Here's how the part is built. I have some questions about the finished solid (model axes, mm). A direction names the side the tool comes from. Give positions to 0.01 mm unless a question says otherwise; leave off trailing zeros. Loops run counter-clockwise (first coordinate to the right, second up) from the corner with the lowest first, then second, coordinate; pieces in that order, holes last. Notation, with made-up numbers: (4, -35.75) -> (47, -35.75) arc R13 ccw to (47, -23.75) -> close; hole circle Ø4 at (7, 39.25). An arc over 180 degrees is marked (long way). Answer in a Markdown table with one row per item. Add a question column.
Item 1: If we section it at C-C (x = 69.5): Write out the boundary of the cut face in (y, z), then the cut area to 3 significant figures.
Item 2: For P1, Ø2, axis at x = 22, z = 36, coming from the +Y side; P2, Ø19, axis at x = 15.5, y = -41.5, coming from the +Z side (3 decimals); P3, Ø20.5, axis at y = 11, z = 26.5, coming from the -X side (3 decimals), each with a flat end and sliding along its axis, tell me the tip position at first contact or that it passes through.
Item 3: If we section it at B-B (y = -44): Write out the boundary of the cut face in (x, z) (3 decimals), then the cut area to 3 significant figures.
Item 4: If we section it at A-A (z = 1): Write out the boundary of the cut face in (x, y) (3 decimals), then the cut area to 3 significant figures.
Item 5: Which directions (+Z, -Z, +X, -X, +Y, -Y) give clear straight access to the entire face, cutting with the end or side of a thin tool? Please do faces 1 (the face through (-1, -1, -9.525)), 2 (the face through (63, 0, 44.542)), 3 (the face through (26.035, 13, 27)), 4 (the face through (48, 25.4, 46)), 5 (the face through (21, -25.4, 35)).
Item 6: If I drill on line 1 (Z direction, x = 65.5, y = -13); line 2 (Y direction, x = 63.5, z = 45.5); line 3 (Y direction, x = 16, z = 33), over which ranges is the centre line in solid material (lowest first)?
```python
from build123d import *

# Parameters (mm, degrees)
F1_DEPTH = 63.5
F0_W     = 25.4
F0_H     = 15.24
F2_DEPTH = 25.4
F3_DEPTH = 25.4
F4_R     = 6.35


with BuildPart() as f1:
    # F0 (on Front) → F1 (new body, symmetric)
    with BuildSketch(Plane.XZ):
        Polygon((41.275, -9.525), (41.275, 9.525), (26.035, 9.525), (-41.275, 9.525), (-41.275, -9.525), align=None)
    extrude(amount=F1_DEPTH, both=True)

    # F0 (on Front) → F2 (join, symmetric)
    with BuildSketch(Plane.XZ):
        with BuildLine():
            Line((26.035, 9.525), (41.275, 9.525))
            Line((41.275, 9.525), (41.275, 43.0532871165))
            ThreePointArc((41.275, 43.0532871165), (41.710954306, 44.1057739147), (42.7634411042, 44.5417282207))
            Line((42.7634411042, 44.5417282207), (58.6539360017, 44.5417282207))
            Line((58.6539360017, 44.5417282207), (58.6539360017, 59.7817282207))
            Line((58.6539360017, 59.7817282207), (42.7634411042, 59.7817282207))
            add(Edge.make_bspline(
                [(42.7634411042, 59.7817282207), (40.0314907438, 59.0712143993), (37.3116085618, 58.3664493175), (34.6130178648, 57.6618922106)],
                knots=[0, 0, 0, 0, 6.2650251323, 6.2650251323, 6.2650251323, 6.2650251323], degree=3))
            ThreePointArc((34.6130178648, 57.6618922106), (28.3380361374, 51.5237318109), (26.035, 43.0532871165))
            Line((26.035, 43.0532871165), (26.035, 9.525))
        make_face()
        with Locations((71.3539360017, 52.1617282207)):
            Rectangle(F0_W, F0_H)
    extrude(amount=F2_DEPTH, both=True)

    # F0 (on Front) → F3 (join)
    with BuildSketch(Plane.XZ):
        with BuildLine():
            Line((-41.275, 9.525), (26.035, 9.525))
            Line((26.035, 9.525), (26.035, 43.0532871165))
            ThreePointArc((26.035, 43.0532871165), (28.3380361374, 51.5237318109), (34.6130178648, 57.6618922106))
            add(Edge.make_bspline(
                [(34.6130178648, 57.6618922106), (-4.8660731715, 47.3545587597), (-39.7882987615, 37.0917367173), (-41.275, 9.525)],
                knots=[6.2650251323, 6.2650251323, 6.2650251323, 6.2650251323, 97.9193459674, 97.9193459674, 97.9193459674, 97.9193459674], degree=3))
        make_face()
    extrude(amount=F3_DEPTH)

    # F4
    f4_edges = [f1.edges().sort_by_distance(p)[0] for p in [
        (41.275, -63.5, 0),
        (-41.275, -63.5, 0),
        (41.275, 63.5, 0),
        (-41.275, 63.5, 0),
    ]]
    fillet(f4_edges, radius=F4_R)


solid = f1.part
```
Recorded:
| question | item | result |
|---|---|---|
| 1 | outline | (-25.4, 44.54) -> (25.4, 44.54) -> (25.4, 59.78) -> (-25.4, 59.78) -> close |
| 1 | area | 774 mm^2 |
| 2 | P1 | stops at y = 0 |
| 2 | P2 | stops at z = 9.525 |
| 2 | P3 | stops at x = 26.035 |
| 3 | outline | (-41.275, -9.525) -> (41.275, -9.525) -> (41.275, 9.525) -> (-41.275, 9.525) -> close |
| 3 | area | 1,570 mm^2 |
| 4 | outline | (-41.275, -57.15) arc R6.35 ccw to (-34.925, -63.5) -> (34.925, -63.5) arc R6.35 ccw to (41.275, -57.15) -> (41.275, 57.15) arc R6.35 ccw to (34.925, 63.5) -> (-34.925, 63.5) arc R6.35 ccw to (-41.275, 57.15) -> close |
| 4 | area | 10,400 mm^2 |
| 5 | face 1 | -Z, +X, -X, +Y, -Y |
| 5 | face 2 | -Z, +X, +Y, -Y |
| 5 | face 3 | +Z, -X, +Y |
| 5 | face 4 | +Z, +X, -X, +Y |
| 5 | face 5 | +Z, +X, -X, -Y |
| 6 | line 1 | z = 44.54 to 59.78 |
| 6 | line 2 | y = -25.4 to 25.4 |
| 6 | line 3 | y = -25.4 to 0 |
